Here's the drawing with two shaded views (mm, measured from the low corner). I have some questions. A direction names the side the tool comes from. Coordinates: 2 decimals unless noted, no trailing zeros. Write each loop counter-clockwise with the first axis right and the second up, starting at its lowest first coordinate (ties: lowest second). Pieces come first, ordered by that corner, then holes.
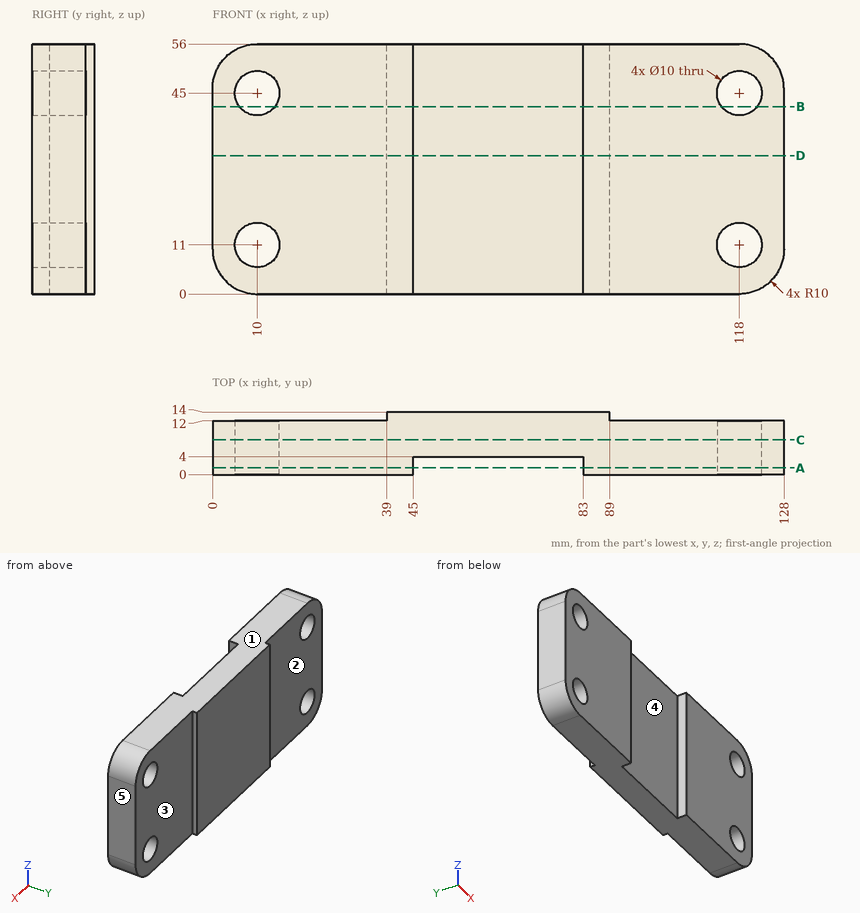
Item 1: If we mould it in two halves opening along X, with no side actions, what happens to the marked faces 3, 4 and 5? For each: released by +X, released by -X, zero draft, split by the parting line, or undercut.
Item 2: If I drill on line 1 along Z through (x, y) = (118, 7.75); line 2 along X through (y, z) = (1.5, 36.5); line 3 along X through (y, z) = (6.5, 13), over which ranges is the centre line in solid material (lowest first)?
Item 3: I want a section at C-C, the plane y = 7.75. List the corners of the cut face in (x, z) for me, then the cut area to 3 significant figures.
Item 4: Will these pins go through, and if not, where does the flat tip stop? pin 1 Ø3 at (y, z) = (12, 48) entering from +X; pin 2 Ø1.6 at (y, z) = (13.5, 40.5) entering from -X; pin 3 Ø19 at (x, z) = (58, 18) entering from -Y.
Item 5: I want a section at B-B, the plane z = 42. List the corners of the cut face in (x, y) for me.
Item 6: I want a section at A-A, the plane y = 1.5. List the corners of the cut face in (x, z) for me.
Item 7: I want a section at D-D, the plane z = 31. List the corners of the cut face in (x, y) for me.
Item 8: Which directions (+Z, -Z, +X, -X, +Y, -Y) give clear straight access to the entire face, cutting with the end or side of a thin tool? Please do the marked faces 1 and 2.
Taken from the geometry:
1. face 3: zero draft
1. face 4: undercut
1. face 5: released by +X
2. line 1: z = 0 to 6, 16 to 40, 50 to 56
2. line 2: x = 0 to 45, 83 to 128
2. line 3: x = 0 to 5.42, 14.58 to 113.42, 122.58 to 128
3. outline: (0, 10) arc R10 ccw to (10, 0) - (118, 0) arc R10 ccw to (128, 10) - (128, 46) arc R10 ccw to (118, 56) - (10, 56) arc R10 ccw to (0, 46) - close; hole circle Ø10 at (10, 11); hole circle Ø10 at (10, 45); hole circle Ø10 at (118, 11); hole circle Ø10 at (118, 45)
3. area: 6,770 mm2
4. pin 1: stops at x = 127.99
4. pin 2: stops at x = 39
4. pin 3: stops at y = 4
5. outline: (0, 0) - (6, 0) - (6, 12) - (0, 12) - close; (14, 0) - (45, 0) - (45, 4) - (83, 4) - (83, 0) - (114, 0) - (114, 12) - (89, 12) - (89, 14) - (39, 14) - (39, 12) - (14, 12) - close; (122, 0) - (128, 0) - (128, 12) - (122, 12) - close
6. outline: (0, 10) arc R10 ccw to (10, 0) - (45, 0) - (45, 56) - (10, 56) arc R10 ccw to (0, 46) - close; (83, 0) - (118, 0) arc R10 ccw to (128, 10) - (128, 46) arc R10 ccw to (118, 56) - (83, 56) - close; hole circle Ø10 at (10, 11); hole circle Ø10 at (10, 45); hole circle Ø10 at (118, 11); hole circle Ø10 at (118, 45)
7. outline: (0, 0) - (45, 0) - (45, 4) - (83, 4) - (83, 0) - (128, 0) - (128, 12) - (89, 12) - (89, 14) - (39, 14) - (39, 12) - (0, 12) - close
8. face 1: +Z, +X, -X, +Y, -Y
8. face 2: +Z, -Z, -X, +Y
